Could you check a few things on this model? Use its own coordinates, in mm. A direction names the side the tool comes from. Round coordinates to 2 decimals unless told otherwise and drop trailing zeros. Write each loop counter-clockwise with the first axis right and the second up, starting at its lowest first coordinate (ties: lowest second). Pieces come first, ordered by that corner, then holes. Notation, with made-up numbers: (-19, 27.5) -> (38, 27.5) arc R14 cw to (38, 49.5) -> close; hole circle Ø1 at (13.25, 79.5). An arc over 180 degrees is marked (long way). Answer in a Markdown table with one row per item. Add a question column.
```python
from build123d import *

# Parameters (mm, degrees)
EXTRUDE_1_DEPTH      = 0.3
EXTRUDE_1_DEPTH_BACK = 0.3


with BuildPart() as part:
    # 草圖1 → 填料-伸長1 (new, two sides: drawn at the far end of the back side and taken through both)
    with BuildSketch(Plane.XY.offset(-EXTRUDE_1_DEPTH_BACK)):
        with BuildLine():
            Line((-3.5, -2.828427125), (-1.75, -0.968245837))
            ThreePointArc((-1.75, -0.968245837), (-1.936491673, -0.5), (-2, 0))
            Line((-2, 0), (-3.4, 0))
            ThreePointArc((-3.4, 0), (-2.697401357, 2.069788859), (-0.879984753, 3.284147809))
            Line((-0.879984753, 3.284147809), (-0.51763809, 1.931851653))
            ThreePointArc((-0.51763809, 1.931851653), (0, 2), (0.51763809, 1.931851653))
            Line((0.51763809, 1.931851653), (0.879984753, 3.284147809))
            ThreePointArc((0.879984753, 3.284147809), (2.697401357, 2.069788859), (3.4, 0))
            Line((3.4, 0), (2, 0))
            ThreePointArc((2, 0), (1.936491673, -0.5), (1.75, -0.968245837))
            Line((1.75, -0.968245837), (3.5, -2.828427125))
            ThreePointArc((3.5, -2.828427125), (0, 4.5), (-3.5, -2.828427125))
        make_face()
    extrude(amount=EXTRUDE_1_DEPTH + EXTRUDE_1_DEPTH_BACK)


solid = part.part
```
(1) Suppose I cut it at B-B, the plane y = 2.25. Please give me the cut outline in (x, z).
(2) Suppose I cut it at A-A, the plane x = -2.25. Please give me the cut outline in (y, z).
(3) On a 3-axis mill with a long thin cutter (end or side, diameter ignored), from which of +Z, -Z, +X, -X, +Y, -Y can I reach the whole of each face in a straight line? I mean faces 1 (the face through (-0.4, 2.2, -0.3)), 2 (the face through (-2.637, -1.911, -0.004)), 3 (the face through (2.68, 2.09, 0)). Say none if no direction works.
(4) Suppose I cut it at D-D, the plane y = 1. Please give me the cut outline in (x, z).
(5) If we mould it in two halves opening along X, with no side actions, what happens to faces 4 (the face through (0.1, 4.5, 0)), 5 (the face through (-0.4, 2.2, 0.3)), 6 (the face through (2.613, -1.885, -0.004))? For each: pulls with the +X half, pulls with the -X half, needs draft (parallel to the pull), parting line crosses it, or undercut.
(6) I need wall thicknesses on L1, parallel to X at y = 1.25, z = 0.1; L2, parallel to X at y = 2.5, z = 0.2; L3, parallel to X at y = 0.5, z = 0.1. Which ranges of each line are inside material? Lowest first, please.
(7) Suppose I cut it at C-C, the plane z = -0.2. Please give me the cut outline in (x, y), then the cut area to 3 significant figures.
Response:
| question | item | result |
|---|---|---|
| 1 | outline | (-3.9, -0.3) -> (-2.55, -0.3) -> (-2.55, 0.3) -> (-3.9, 0.3) -> close; (-0.6, -0.3) -> (0.6, -0.3) -> (0.6, 0.3) -> (-0.6, 0.3) -> close; (2.55, -0.3) -> (3.9, -0.3) -> (3.9, 0.3) -> (2.55, 0.3) -> close |
| 2 | outline | (-1.5, -0.3) -> (0, -0.3) -> (0, 0.3) -> (-1.5, 0.3) -> close; (2.55, -0.3) -> (3.9, -0.3) -> (3.9, 0.3) -> (2.55, 0.3) -> close |
| 3 | face 1 | -Z, +X, -X, +Y, -Y |
| 3 | face 2 | +Z, -Z, -Y |
| 3 | face 3 | +Z, -Z |
| 4 | outline | (-4.39, -0.3) -> (-3.25, -0.3) -> (-3.25, 0.3) -> (-4.39, 0.3) -> close; (3.25, -0.3) -> (4.39, -0.3) -> (4.39, 0.3) -> (3.25, 0.3) -> close |
| 5 | face 4 | parting line crosses it |
| 5 | face 5 | needs draft |
| 5 | face 6 | undercut |
| 6 | L1 | -4.32 to -3.16, 3.16 to 4.32 |
| 6 | L2 | -3.74 to -2.3, -0.67 to 0.67, 2.3 to 3.74 |
| 6 | L3 | -4.47 to -3.36, 3.36 to 4.47 |
| 7 | outline | (-3.5, -2.83) -> (-1.75, -0.97) arc R2 cw to (-2, 0) -> (-3.4, 0) arc R3.4 cw to (-0.88, 3.28) -> (-0.52, 1.93) arc R2 cw to (0.52, 1.93) -> (0.88, 3.28) arc R3.4 cw to (3.4, 0) -> (2, 0) arc R2 cw to (1.75, -0.97) -> (3.5, -2.83) arc R4.5 ccw (long way) to start |
| 7 | area | 25.8 mm² |
